from build123d import *

# Parameters (mm, degrees)
SKETCH1_R           = 1.4
BOSS_EXTRUDE1_DEPTH = 4
SKETCH2_R           = 1.521670414
SKETCH2_R_2         = 1.472584271
CUT_EXTRUDE1_DEPTH  = 10
SKETCH3_R           = 1.4
CUT_EXTRUDE2_DEPTH  = 10


with BuildPart() as part:
    # Sketch1 → Boss-Extrude1 (new body)
    with BuildSketch(Plane.XY):
        with BuildLine():
            Line((-15.500688459, 45.016091721), (-11.000688459, -8.006682704))
            ThreePointArc((-11.000688459, -8.006682704), (-5.500688459, -13.506682704), (-0.000688459, -8.006682704))
            Line((-0.000688459, -8.006682704), (4.499311541, 45.016091721))
            ThreePointArc((4.499311541, 45.016091721), (-5.500688459, 55.016091721), (-15.500688459, 45.016091721))
        make_face()
        with Locations((-5.500688459, -8.006682704)):
            Circle(SKETCH1_R, mode=Mode.SUBTRACT)
        with Locations((-5.500688459, 45.016091721)):
            Circle(SKETCH1_R, mode=Mode.SUBTRACT)
        with Locations((1.499311541, 45.016091721)):
            Circle(SKETCH1_R, mode=Mode.SUBTRACT)
        with Locations((-12.500688459, 45.016091721)):
            Circle(SKETCH1_R, mode=Mode.SUBTRACT)
    extrude(amount=BOSS_EXTRUDE1_DEPTH)

    # Sketch2 → Cut-Extrude1 (cut)
    with BuildSketch(Plane.XY.offset(4)):
        with Locations((-5.500688459, 38.016091721)):
            Circle(SKETCH2_R)
        with Locations((-5.500688459, 52.016091721)):
            Circle(SKETCH2_R_2)
    extrude(amount=-CUT_EXTRUDE1_DEPTH, mode=Mode.SUBTRACT)

    # Sketch3 → Cut-Extrude2 (cut)
    with BuildSketch(Plane.XY.offset(4)):
        with Locations((-5.500688459, 25.016091721)):
            Circle(SKETCH3_R)
    extrude(amount=-CUT_EXTRUDE2_DEPTH, mode=Mode.SUBTRACT)


solid = part.part
Check sheet for the modelled part. Datum: model origin and axes. Units: mm. Round coordinates to 2 decimals unless told otherwise and drop trailing zeros. Loops run counter-clockwise (first coordinate to the right, second up) from the corner with the lowest first, then second, coordinate; pieces in that order, holes last. Notation, with made-up numbers: (19.5, -19.75) -> (33.5, -19.75) arc R5 cw to (33.5, -14.75) -> close; hole circle Ø4 at (23, 82). An arc over 180 degrees is marked (long way). Put each result on its own line as item: value. Start each with the question number.
1. Section check D-D (y = 18.5). Enter the section's corners in (x, z).
2. Scan lines: probe 1 along Y at (x, z) = (-5, 2.7); probe 2 along Y at (x, z) = (-5.25, 0.5) (3 decimals); probe 3 along X at (y, z) = (37, 1.7). Record each from-to range of solid material in increasing order.
3. Section check A-A (x = -12.5). Enter the section's corners in (y, z).
4. Gauge pin test, flat ends, axial feed: pin 1 (4.5 mm diameter, centred on x = -5.5, y = -8.01, fed in from +Z); pin 2 (2 mm diameter, centred on x = 1.5, y = 45.02, fed in from +Z); pin 3 (1 mm diameter, centred on y = 35, z = 1.5, fed in from +X). Record the tip position at first contact, or that the pin passes through.
5. Draft check along X on faces 1 (the face through (2.218, 18.134, 1.972)), 2 (the face through (-4.71, 53.26, 2.03)), 3 (the face through (-5.281, 55.014, 1.972)). Enter one of: +X half, -X half, draft (parallel to the pull), parting line (faces both ways), or undercut.
6. Section check B-B (z = 2.5). Enter the section's corners in (x, y), plus the area to 3 significant figures.
7. Section check C-C (x = -6). Enter the section's corners in (y, z), plus the area to 3 significant figures.
Findings:
1. outline: (-13.25, 0) -> (2.25, 0) -> (2.25, 4) -> (-13.25, 4) -> close
2. probe 1: y = -13.48 to -9.31, -6.7 to 23.71, 26.32 to 36.58, 39.45 to 43.71, 46.32 to 50.63, 53.4 to 55
2. probe 2: y = -13.501 to -9.384, -6.629 to 23.639, 26.393 to 36.515, 39.517 to 43.639, 46.393 to 50.565, 53.467 to 55.013
2. probe 3: x = -14.82 to -6.63, -4.37 to 3.82
3. outline: (9.66, 0) -> (43.62, 0) -> (43.62, 4) -> (9.66, 4) -> close; (46.42, 0) -> (52.16, 0) -> (52.16, 4) -> (46.42, 4) -> close
4. pin 1: stops at z = 4
4. pin 2: passes through
4. pin 3: stops at x = 3.69
5. face 1: +X half
5. face 2: undercut
5. face 3: parting line
6. outline: (-15.5, 45.02) -> (-11, -8.01) arc R5.5 ccw to (0, -8.01) -> (4.5, 45.02) arc R10 ccw to start; hole circle Ø2.8 at (-12.5, 45.02); hole circle Ø3.04 at (-5.5, 38.02); hole circle Ø2.95 at (-5.5, 52.02); hole circle Ø2.8 at (-5.5, -8.01); hole circle Ø2.8 at (-5.5, 25.02); hole circle Ø2.8 at (-5.5, 45.02); hole circle Ø2.8 at (1.5, 45.02)
6. area: 982 mm^2
7. outline: (-13.48, 0) -> (-9.31, 0) -> (-9.31, 4) -> (-13.48, 4) -> close; (-6.7, 0) -> (23.71, 0) -> (23.71, 4) -> (-6.7, 4) -> close; (26.32, 0) -> (36.58, 0) -> (36.58, 4) -> (26.32, 4) -> close; (39.45, 0) -> (43.71, 0) -> (43.71, 4) -> (39.45, 4) -> close; (46.32, 0) -> (50.63, 0) -> (50.63, 4) -> (46.32, 4) -> close; (53.4, 0) -> (55, 0) -> (55, 4) -> (53.4, 4) -> close
7. area: 220 mm^2
